from build123d import *

# Parameters (mm, degrees)
F0_R     = 25
F1_DEPTH = 40
F2_W     = 20
F2_H     = 40
F3_DEPTH = 100
F4_R     = 15
F5_DEPTH = 43


with BuildPart() as f1:
    # F0 (on Top) → F1 (new body)
    with BuildSketch(Plane.XY):
        Circle(F0_R)
    extrude(amount=F1_DEPTH)

    # F2 (on Front) → F3 (join)
    with BuildSketch(Plane.XZ):
        with Locations((0, 20)):
            Rectangle(F2_W, F2_H)
    extrude(amount=-F3_DEPTH)

    # F4 (on face) → F5 (cut)
    with BuildSketch(Plane.XY.offset(40)):
        Circle(F4_R)
    extrude(amount=-F5_DEPTH, mode=Mode.SUBTRACT)


solid = f1.part
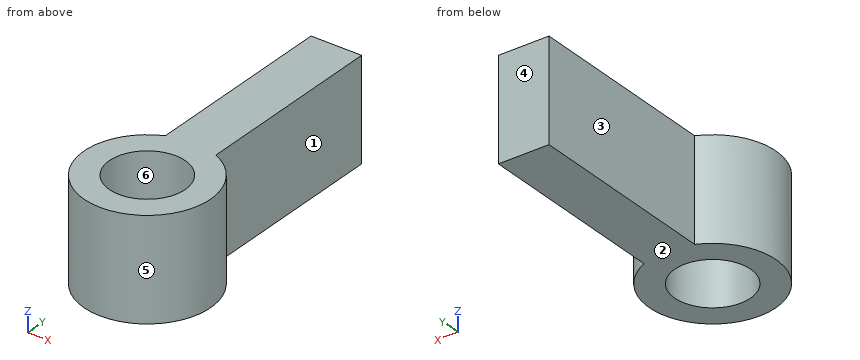
Read the model definition and answer for the solid it produces. Units are mm, in the model's axes. Face numbers are marked on the shaded views. A direction names the side the tool comes from. Give positions to 0.01 mm unless a question says otherwise; leave off trailing zeros. Write each loop counter-clockwise with the first axis right and the second up, starting at its lowest first coordinate (ties: lowest second). Pieces come first, ordered by that corner, then holes. Notation, with made-up numbers: (22, 47.25) - (50, 47.25) arc R32 cw to (50, 86.25) - close; hole circle Ø5 at (18, -20.75). An arc over 180 degrees is marked (long way). Use CSV: the item, a comma, the result in double quotes. Start each with the question number.
(1) For the marked faces 1, 2 and 3, determine the directions among +Z, -Z, +X, -X, +Y, -Y from which every point of the face is accessible in a straight line to the end or side of a thin tool.
(2) Consider line 1 along Y through (x, z) = (0, 25); line 2 along X through (y, z) = (41, 29); line 3 along Y through (x, z) = (-9.5, 18.5). Determine where each line is inside the solid, lowest interval first.
(3) Find section C-C (z = 5). Give the vertices of the cut face in (x, y), plus the area to 3 significant figures.
(4) Determine the mould class of the marked faces 4, 5 and 6 for opening direction X: +X half, -X half, draft (parallel to the pull), parting line (faces both ways), or undercut.
(5) Find section A-A (x = 0). Give the vertices of the cut face in (y, z), plus the area to 3 significant figures.
(6) Find section D-D (x = 18). Give the vertices of the cut face in (y, z).
(7) Given P1, Ø4, axis at x = 5.5, z = 30, coming from the -Y side; P2, Ø3, axis at y = 65, z = 21.5, coming from the -X side; P3, Ø1.5, axis at y = 6.5, z = 23.5, coming from the +X side; P4, Ø2, axis at x = 8, y = 63, coming from the -Z side, each flat-ended and moving along its own axis, determine where each tip first touches the part or whether it passes through.
(8) Find section B-B (y = 0). Give the vertices of the cut face in (x, z), plus the area to 3 significant figures.
Findings below:
1,face 1,"+Z, -Z, +X, +Y"
1,face 2,"-Z, +X, -X, +Y, -Y"
1,face 3,"+Z, -Z, -X, +Y"
2,line 1,"-25 to -15, 15 to 100"
2,line 2,"-10 to 10"
2,line 3,"-23.12 to -11.61, 11.61 to 100"
3,outline,"(-10, 22.91) arc R25 ccw (long way) to (10, 22.91) - (10, 100) - (-10, 100) - close; hole circle Ø30 at (0, 0)"
3,area,"2,770 mm2"
4,face 4,"draft"
4,face 5,"parting line"
4,face 6,"undercut"
5,outline,"(-25, 0) - (-15, 0) - (-15, 40) - (-25, 40) - close; (15, 0) - (100, 0) - (100, 40) - (15, 40) - close"
5,area,"3,800 mm2"
6,outline,"(-17.35, 0) - (17.35, 0) - (17.35, 40) - (-17.35, 40) - close"
7,P1,"y = -24.75"
7,P2,"x = -10"
7,P3,"x = 24.33"
7,P4,"z = 0"
8,outline,"(-25, 0) - (-15, 0) - (-15, 40) - (-25, 40) - close; (15, 0) - (25, 0) - (25, 40) - (15, 40) - close"
8,area,"800 mm2"
